Design review of the part built by this model. Coordinates are the model's own, in mm. Face numbers are marked on the shaded views. A direction names the side the tool comes from. Coordinates: 2 decimals unless noted, no trailing zeros. Write each loop counter-clockwise with the first axis right and the second up, starting at its lowest first coordinate (ties: lowest second). Pieces come first, ordered by that corner, then holes. Notation, with made-up numbers: (16.5, 87.5) - (24.5, 87.5) arc R19 cw to (24.5, 110.5) - close; hole circle Ø2 at (26, -24). An arc over 180 degrees is marked (long way). Answer as CSV lines item,"result". Start each with the question number.
Q1. We need section C-C (z = 5.25). Write out the cut boundary in (x, y).
Q2. We need section D-D (x = -3). Write out the cut boundary in (y, z), plus the area to 3 significant figures.
Q3. For line 1 along Z through (x, y) = (-2, 2.5); line 2 along X through (y, z) = (-2, 7.75); line 3 along Y through (x, z) = (-1.5, 9.5), list the stretches that pass through material, from the lowest coordinate up. Write a range as [from, to].
Q4. We need section B-B (y = 0.5). Write out the cut boundary in (x, z).
Q5. Machinability: for the marked faces 1 and 2, which of the approach directions +Z, -Z, +X, -X, +Y, -Y give a long, thin tool a straight path to every point of the face, cutting with its end or side? Answer none if there is none.
Q6. We need section A-A (x = 0). Write out the cut boundary in (y, z), plus the area to 3 significant figures.
Q7. Clearance check with flat-ended pins moving along their axes: pin 1 (3 mm diameter, centred on y = 1.5, z = 6, fed in from +X); pin 2 (1 mm diameter, centred on x = -2.5, z = 11.5, fed in from -Y); pin 3 (4 mm diameter, centred on x = -1.5, z = 13.5, fed in from -Y). State where each tip first meets the part, or that it passes through.
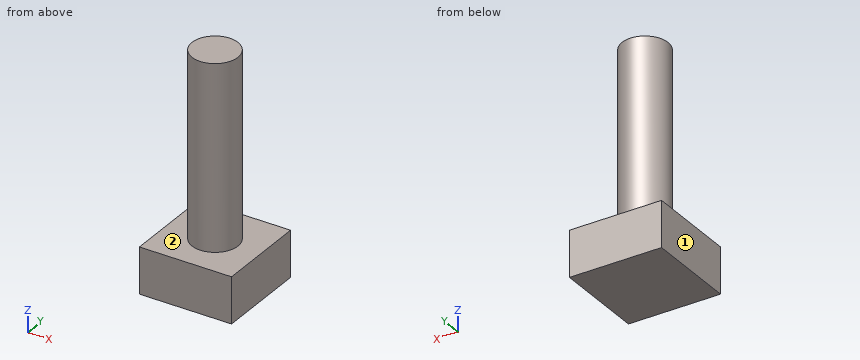
from build123d import *

# Parameters (mm, degrees)
F0_R     = 2.5
F1_DEPTH = 20
F2_W     = 10
F2_H     = 10
F3_DEPTH = 5


with BuildPart() as f1:
    # F0 (on Top) → F1 (new body)
    with BuildSketch(Plane.XY):
        Circle(F0_R)
    extrude(amount=F1_DEPTH)

    # F2 (on face) → F3 (join)
    with BuildSketch(Plane(origin=(0, 0, 0), x_dir=(1, 0, 0), z_dir=(0, 0, -1))):
        Rectangle(F2_W, F2_H)
    extrude(amount=F3_DEPTH)


solid = f1.part
Results list:
1,outline,"circle Ø5 at (0, 0)"
2,outline,"(-5, -5) - (5, -5) - (5, 0) - (-5, 0) - close"
2,area,"50.0 mm2"
3,line 1,"z = [-5, 0]"
3,line 2,"x = [-1.5, 1.5]"
3,line 3,"y = [-2, 2]"
4,outline,"(-5, -5) - (5, -5) - (5, 0) - (2.45, 0) - (2.45, 20) - (-2.45, 20) - (-2.45, 0) - (-5, 0) - close"
5,face 1,"+Z, -Z, -X, +Y, -Y"
5,face 2,"+Z"
6,outline,"(-5, -5) - (5, -5) - (5, 0) - (2.5, 0) - (2.5, 20) - (-2.5, 20) - (-2.5, 0) - (-5, 0) - close"
6,area,"150 mm2"
7,pin 1,"stops at x = 2.5"
7,pin 2,"stops at y = -1.5"
7,pin 3,"stops at y = -2.5"
